```python
from build123d import *

# Parameters (mm, degrees)
F0_W     = 317.5
F0_H     = 76.2
F1_DEPTH = 25.4
F3_DEPTH = 50.8
F5_DEPTH = 508


with BuildPart() as f1:
    # F0 (on Front) → F1 (new body)
    with BuildSketch(Plane.XZ):
        with Locations((24.531897, 23.258603)):
            Rectangle(F0_W, F0_H)
    extrude(amount=F1_DEPTH)

    # F2 (on face) → F3 (cut)
    with BuildSketch(Plane.XZ.offset(25.4)):
        Polygon((-134.218103, -14.841397), (-108.818103, -14.841397), (-41.616019, 61.358603), (-134.218103, 61.358603), align=None)
        Polygon((90.679814, 61.358603), (157.881897, -14.841397), (183.281897, -14.841397), (183.281897, 61.358603), align=None)
    extrude(amount=-F3_DEPTH, mode=Mode.SUBTRACT)

    # F4 (on face) → F5 (cut)
    with BuildSketch(Plane.XZ.offset(25.4)):
        with BuildLine():
            Line((-83.418103, -14.841397), (132.481897, -14.841397))
            ThreePointArc((132.481897, -14.841397), (24.531897, 4.208603), (-83.418103, -14.841397))
        make_face()
    extrude(amount=-F5_DEPTH, mode=Mode.SUBTRACT)


solid = f1.part
```
Geometry check sheet. Reference: the model listing, model coordinates, mm. Round coordinates to 2 decimals unless told otherwise and drop trailing zeros. Loops run counter-clockwise (first coordinate to the right, second up) from the corner with the lowest first, then second, coordinate; pieces in that order, holes last. Notation, with made-up numbers: M 58.5,26.5 L 111.5,26.5 A19 cw 111.5,47.5 Z; hole C 85.5,9.25 d7. An arc over 180 degrees is marked long. Return JSON: item names as keys, results as strings. Group by question number.
(1) Section check D-D, the plane z = 26.5. Enter the section's corners in (x, y), and give its area (3 significant figures).
(2) Section check B-B, the plane z = -3. Enter the section's corners in (x, y), and give its area (3 significant figures).
(3) Section check C-C, the plane x = -79. Enter the section's corners in (y, z), and give its area (3 significant figures).
(4) Section check A-A, the plane y = -5.75. Enter the section's corners in (x, z).
(5) Mould release check, pull along X, two halves, no side actions. Record for faces 1 (the face through (-75.687, -12.878, 22.725)), 2 (the face through (26.074, -12.878, 4.205)), 3 (the face through (24, -13, 61.359)), 4 (the face through (123.81, -12.88, 23.79)): pulls with the +X half, pulls with the -X half, needs draft (parallel to the pull), parting line crosses it, or undercut.
(6) Scan lines: line 1 along X through (y, z) = (-22.5, 50); line 2 along X through (y, z) = (-5.5, 27.5); line 3 along Z through (x, y) = (-51, -1.75). Record each from-to range of solid material in increasing order. Write a range as [from, to].
(7) Go/stop test with flat-tipped pins: pin 1 (2 mm diameter, centred on x = -9, z = 2, fed in from -Y); pin 2 (2 mm diameter, centred on y = -16, z = 20.5, fed in from -X); pin 3 (10 mm diameter, centred on y = -10, z = 17, fed in from +X); pin 4 (2 mm diameter, centred on y = -8, z = 33, fed in from -X). Record where each tip stops, or that it passes through.
Data:
{
 "1": {"outline": "M -72.36,-25.4 L 121.42,-25.4 L 121.42,0 L -72.36,0 Z", "area": "4,920 mm²"},
 "2": {"outline": "M -98.37,-25.4 L -42.51,-25.4 L -42.51,0 L -98.37,0 Z; M 91.58,-25.4 L 147.44,-25.4 L 147.44,0 L 91.58,0 Z", "area": "2,840 mm²"},
 "3": {"outline": "M -25.4,-13.27 L 0,-13.27 L 0,18.97 L -25.4,18.97 Z", "area": "819 mm²"},
 "4": {"outline": "M -108.82,-14.84 L -83.42,-14.84 A315.38 cw 132.48,-14.84 L 157.88,-14.84 L 90.68,61.36 L -41.62,61.36 Z"},
 "5": {"face 1": "pulls with the -X half", "face 2": "undercut", "face 3": "needs draft", "face 4": "pulls with the +X half"},
 "6": {"line 1": "[-51.63, 100.7]", "line 2": "[-71.48, 120.54]", "line 3": "[-4.97, 50.72]"},
 "7": {"pin 1": "y = -25.4", "pin 2": "x = -78.53", "pin 3": "x = 134.21", "pin 4": "x = -67.51"}
}
